Read the model definition and answer for the solid it produces. Units are mm, in the model's axes. A direction names the side the tool comes from. Coordinates: 2 decimals unless noted, no trailing zeros. Order: outer loops, then holes, each group sorted by start corner. A loop starts at its lowest first (then second) coordinate and runs counter-clockwise, first axis right, second up.
from build123d import *

# Parameters (mm, degrees)
SKETCH_1_W          = 80
SKETCH_1_H          = 40
EXTRUDE_1_DEPTH     = 1000
SKETCH_2_W          = 400
SKETCH_2_H          = 40
EXTRUDE_2_DEPTH     = 40
SKETCH_3_W          = 400
SKETCH_3_H          = 40
EXTRUDE_3_DEPTH     = 40
CUT_EXTRUDE_1_DEPTH = 121


with BuildPart() as part:
    # 草图1 → 凸台-拉伸1 (new body)
    with BuildSketch(Plane(origin=(0, 0, 0), x_dir=(1, 0, 0), z_dir=(0, 1, 0))):
        with Locations((40, -20)):
            Rectangle(SKETCH_1_W, SKETCH_1_H)
    extrude(amount=EXTRUDE_1_DEPTH)

    # 草图2 → 凸台-拉伸2 (add)
    with BuildSketch(Plane.XY.offset(40)):
        with Locations((40, 980)):
            Rectangle(SKETCH_2_W, SKETCH_2_H)
    extrude(amount=EXTRUDE_2_DEPTH)

    # 草图3 → 凸台-拉伸3 (add)
    with BuildSketch(Plane(origin=(0, 0, 0), x_dir=(-1, 0, 0), z_dir=(0, 0, -1))):
        with Locations((-40, 980)):
            Rectangle(SKETCH_3_W, SKETCH_3_H)
    extrude(amount=EXTRUDE_3_DEPTH)

    # 草图4 → 切除-拉伸1 (cut, through all)
    with BuildSketch(Plane.XY.offset(80)):
        Polygon((-160, 1000), (-120, 960), (-160, 960), align=None)
        Polygon((240, 1000), (200, 960), (240, 960), align=None)
    extrude(amount=-CUT_EXTRUDE_1_DEPTH, mode=Mode.SUBTRACT)


solid = part.part
Q1. Straight lines are drawn through the part: L1, parallel to X at y = 698.5, z = 3; L2, parallel to Y at x = 193.5, z = 65.5; L3, parallel to Z at x = 6, y = 746. For each, find the intervals that lie inside material, in ascending order.
Q2. The part is cut by section B-B, the plane x = 28. Determine the outline of the cut face in (y, z), then the cut area to 3 significant figures.
Q3. The part is cut by section D-D, the plane z = 17.5. Determine the outline of the cut face in (x, y).
Q4. Determine the mould class of faces 1 (the flat face through (220, 980, 60)), 2 (the flat face through (143, 980, 0)), 3 (the flat face through (37, 980, 80)) for opening direction Z: +Z half, -Z half, draft (parallel to the pull), parting line (faces both ways), or undercut.
Q5. The part is cut by section C-C, the plane y = 372.5. Determine the outline of the cut face in (x, z).
Q6. Each of these flat-tipped pins is pushed along its axis until it touches: P1, Ø2, axis at x = 153.5, z = -15, coming from the -Y side; P2, Ø2, axis at x = 30, y = 678.5, coming from the -Z side; P3, Ø12, axis at y = 453, z = 15, coming from the -X side. Where does it stop, or does it pass through?
Q7. Which of the six approach directions +Z, -Z, +X, -X, +Y, -Y give full straight-line access (tool end or side, diameter ignored) to faces 4 (the flat face through (-61, 980, 0)), 5 (the flat face through (141, 980, 40)), 6 (the flat face through (38, 960, 60)), 7 (the flat face through (39, 473, 0))?
Q8. The part is cut by section A-A, the plane x = 211. Determine the outline of the cut face in (y, z).
Computed values:
1. L1: x = 0 to 80
1. L2: y = 960 to 1000
1. L3: z = 0 to 40
2. outline: (0, 0) - (960, 0) - (960, -40) - (1000, -40) - (1000, 80) - (960, 80) - (960, 40) - (0, 40) - close
2. area: 43,200 mm2
3. outline: (0, 0) - (80, 0) - (80, 1000) - (0, 1000) - close
4. face 1: draft
4. face 2: undercut
4. face 3: +Z half
5. outline: (0, 0) - (80, 0) - (80, 40) - (0, 40) - close
6. P1: stops at y = 960
6. P2: stops at z = 0
6. P3: stops at x = 0
7. face 4: -X, +Y, -Y
7. face 5: +X, +Y, -Y
7. face 6: +Z, +X, -X, -Y
7. face 7: -Z, +X, -X, -Y
8. outline: (971, -40) - (1000, -40) - (1000, 0) - (971, 0) - close; (971, 40) - (1000, 40) - (1000, 80) - (971, 80) - close
